```python
from build123d import *

# Parameters (mm, degrees)
F1_DEPTH = 12


with BuildPart() as f1:
    # F0 (on Right) → F1 (new body)
    with BuildSketch(Plane.YZ):
        with BuildLine():
            Line((0, 12), (0, 0))
            Line((0, 0), (54, 0))
            ThreePointArc((54, 0), (58.242641, 1.757359), (60, 6))
            ThreePointArc((60, 6), (58.242641, 10.242641), (54, 12))
            Line((54, 12), (0, 12))
        make_face()
    extrude(amount=F1_DEPTH)


solid = f1.part
```
Verification items for the finished model (mm, model axes). Round coordinates to 2 decimals unless told otherwise and drop trailing zeros. Order: outer loops, then holes, each group sorted by start corner. A loop starts at its lowest first (then second) coordinate and runs counter-clockwise, first axis right, second up.
1) Cross-section at B-B, the plane z = 2.5. Record the cut outline in (x, y), plus the area to 3 significant figures.
Geometry says:
outline: (0, 0) - (12, 0) - (12, 58.87) - (0, 58.87) - close
area: 706 mm2
2) Material ranges on line 1 (Y direction, x = 3.5, z = 1.25); line 2 (Y direction, x = 2, z = 8.5); line 3 (Z direction, x = 8.5, y = 56), recorded low to high.
Geometry says:
line 1: y = 0 to 57.67
line 2: y = 0 to 59.45
line 3: z = 0.34 to 11.66
3) Cross-section at A-A, the plane x = 4.5. Record the cut outline in (y, z), plus the area to 3 significant figures.
Geometry says:
outline: (0, 0) - (54, 0) arc R6 ccw to (60, 6) arc R6 ccw to (54, 12) - (0, 12) - close
area: 705 mm2
4) Cross-section at C-C, the plane z = 10. Record the cut outline in (x, y).
Geometry says:
outline: (0, 0) - (12, 0) - (12, 58.47) - (0, 58.47) - close
5) Depth check by flat-ended pin: pin 1 (5 mm diameter, centred on y = 22.5, z = 7.5, fed in from -X). Enter the tip coordinate at first touch or a pass-through.
Geometry says:
pin 1: stops at x = 0
